from build123d import *

# Parameters (mm, degrees)
SKETCH1_W                = 98
SKETCH1_H                = 63
BOSS_EXTRUDE1_DEPTH      = 12
CUT_EXTRUDE1_REACH       = 61.475
SKETCH2_R                = 10
SKETCH2_R_2              = 6.5
SKETCH2_R_3              = 2.5
CUT_EXTRUDE2_REACH       = 61.475
SKETCH3_W                = 34
SKETCH3_H                = 12
F_5_0_5_DIAMETER_HOLE1_D = 5
CUT_EXTRUDE3_REACH       = 61.475
SKETCH11_W               = 25
SKETCH11_H               = 16
CUT_EXTRUDE4_REACH       = 61.475
FILLET1_R                = 2
CUT_EXTRUDE7_DEPTH       = 8
CUT_EXTRUDE8_DEPTH       = 6.5


with BuildPart() as part:
    # Sketch1 → Boss-Extrude1 (new body)
    with BuildSketch(Plane(origin=(0, 0, 0), x_dir=(1, 0, 0), z_dir=(0, 1, 0))):
        Rectangle(SKETCH1_W, SKETCH1_H)
    extrude(amount=BOSS_EXTRUDE1_DEPTH)

    # Sketch2 → Cut-Extrude1 (cut, up to next)
    with BuildSketch(Plane(origin=(0, 12, 0), x_dir=(1, 0, 0), z_dir=(0, 1, 0)), mode=Mode.PRIVATE) as cut_extrude1_sk1:
        with Locations(Location((0, 16.5, 0), (0, 0, 270))):
            Circle(SKETCH2_R)
    cut_extrude1_tool1 = extrude(cut_extrude1_sk1.sketch, amount=-CUT_EXTRUDE1_REACH, mode=Mode.PRIVATE) & part.part
    # Sketch2 → Cut-Extrude1 (cut, up to next)
    with BuildSketch(Plane(origin=(0, 12, 0), x_dir=(1, 0, 0), z_dir=(0, 1, 0)), mode=Mode.PRIVATE) as cut_extrude1_sk2:
        with Locations(Location((-28, -4.5, 0), (0, 0, 270))):
            Circle(SKETCH2_R_2)
    cut_extrude1_tool2 = extrude(cut_extrude1_sk2.sketch, amount=-CUT_EXTRUDE1_REACH, mode=Mode.PRIVATE) & part.part
    # Sketch2 → Cut-Extrude1 (cut, up to next)
    with BuildSketch(Plane(origin=(0, 12, 0), x_dir=(1, 0, 0), z_dir=(0, 1, 0)), mode=Mode.PRIVATE) as cut_extrude1_sk3:
        with Locations(Location((28, -4.5, 0), (0, 0, 270))):
            Circle(SKETCH2_R_2)
    cut_extrude1_tool3 = extrude(cut_extrude1_sk3.sketch, amount=-CUT_EXTRUDE1_REACH, mode=Mode.PRIVATE) & part.part
    # Sketch2 → Cut-Extrude1 (cut, up to next)
    with BuildSketch(Plane(origin=(0, 12, 0), x_dir=(1, 0, 0), z_dir=(0, 1, 0)), mode=Mode.PRIVATE) as cut_extrude1_sk4:
        with Locations(Location((-15, 16.5, 0), (0, 0, 270))):
            Circle(SKETCH2_R_3)
    cut_extrude1_tool4 = extrude(cut_extrude1_sk4.sketch, amount=-CUT_EXTRUDE1_REACH, mode=Mode.PRIVATE) & part.part
    # Sketch2 → Cut-Extrude1 (cut, up to next)
    with BuildSketch(Plane(origin=(0, 12, 0), x_dir=(1, 0, 0), z_dir=(0, 1, 0)), mode=Mode.PRIVATE) as cut_extrude1_sk5:
        with Locations(Location((15, 16.5, 0), (0, 0, 270))):
            Circle(SKETCH2_R_3)
    cut_extrude1_tool5 = extrude(cut_extrude1_sk5.sketch, amount=-CUT_EXTRUDE1_REACH, mode=Mode.PRIVATE) & part.part
    add(cut_extrude1_tool1.solids().sort_by_distance((0, 12, -16.5))[0], mode=Mode.SUBTRACT)
    add(cut_extrude1_tool2.solids().sort_by_distance((-28, 12, 4.5))[0], mode=Mode.SUBTRACT)
    add(cut_extrude1_tool3.solids().sort_by_distance((28, 12, 4.5))[0], mode=Mode.SUBTRACT)
    add(cut_extrude1_tool4.solids().sort_by_distance((-15, 12, -16.5))[0], mode=Mode.SUBTRACT)
    add(cut_extrude1_tool5.solids().sort_by_distance((15, 12, -16.5))[0], mode=Mode.SUBTRACT)

    # Sketch3 → Cut-Extrude2 (cut, up to next)
    with BuildSketch(Plane(origin=(0, 12, 0), x_dir=(1, 0, 0), z_dir=(0, 1, 0)), mode=Mode.PRIVATE) as cut_extrude2_sk1:
        with Locations((0, -25.5)):
            Rectangle(SKETCH3_W, SKETCH3_H)
    cut_extrude2_tool1 = extrude(cut_extrude2_sk1.sketch, amount=-CUT_EXTRUDE2_REACH, mode=Mode.PRIVATE) & part.part
    add(cut_extrude2_tool1.solids().sort_by_distance((0, 12, 25.5))[0], mode=Mode.SUBTRACT)

    # Ø5.0 (5) Diameter Hole1 (through all)
    with Locations(Plane(origin=(0, 12, 0), x_dir=(-1, 0, 0), z_dir=(0, 1, 0))):
        with Locations((28, 23.5), (-28, 23.5)):
            Hole(F_5_0_5_DIAMETER_HOLE1_D / 2)

    # Sketch11 → Cut-Extrude3 (cut, up to next)
    with BuildSketch(Plane(origin=(0, 12, 0), x_dir=(-1, 0, 0), z_dir=(0, 1, 0)), mode=Mode.PRIVATE) as cut_extrude3_sk1:
        with Locations((36.5, -23.5)):
            Rectangle(SKETCH11_W, SKETCH11_H)
    cut_extrude3_tool1 = extrude(cut_extrude3_sk1.sketch, amount=-CUT_EXTRUDE3_REACH, mode=Mode.PRIVATE) & part.part
    cut_extrude3 = cut_extrude3_tool1.solids().sort_by_distance((-36.5, 12, -23.5))[0]
    add(cut_extrude3, mode=Mode.SUBTRACT)

    # Mirror1: Cut-Extrude3 across plane
    add(cut_extrude3.mirror(Plane(origin=(0, 0, 0), x_dir=(0, 0, 1), z_dir=(1, 0, 0))), mode=Mode.SUBTRACT)

    # Sketch12 → Cut-Extrude4 (cut, up to next)
    with BuildSketch(Plane(origin=(0, 12, 0), x_dir=(1, 0, 0), z_dir=(0, 1, 0)), mode=Mode.PRIVATE) as cut_extrude4_sk1:
        with BuildLine():
            Line((-17, -19.5), (-13, -19.5))
            ThreePointArc((-13, -19.5), (-15, -17.5), (-17, -19.5))
        make_face()
    cut_extrude4_tool1 = extrude(cut_extrude4_sk1.sketch, amount=-CUT_EXTRUDE4_REACH, mode=Mode.PRIVATE) & part.part
    # Sketch12 → Cut-Extrude4 (cut, up to next)
    with BuildSketch(Plane(origin=(0, 12, 0), x_dir=(1, 0, 0), z_dir=(0, 1, 0)), mode=Mode.PRIVATE) as cut_extrude4_sk2:
        with BuildLine():
            Line((13, -19.5), (17, -19.5))
            ThreePointArc((17, -19.5), (15, -17.5), (13, -19.5))
        make_face()
    cut_extrude4_tool2 = extrude(cut_extrude4_sk2.sketch, amount=-CUT_EXTRUDE4_REACH, mode=Mode.PRIVATE) & part.part
    add(cut_extrude4_tool1.solids().sort_by_distance((-15, 12, 18.651174))[0], mode=Mode.SUBTRACT)
    add(cut_extrude4_tool2.solids().sort_by_distance((15, 12, 18.651174))[0], mode=Mode.SUBTRACT)

    # Fillet1
    fillet1_edges = [part.edges().sort_by_distance(p)[0] for p in [
        (-49, 6, -15.5),
        (-24, 6, -31.5),
        (-24, 6, -15.5),
        (49, 6, -15.5),
        (24, 6, -15.5),
        (24, 6, -31.5),
    ]]
    fillet(fillet1_edges, radius=FILLET1_R)

    # Sketch18 → Cut-Extrude7 (cut)
    with BuildSketch(Plane(origin=(-30.447133355, 0, 87.682451642), x_dir=(1, 0, 0), z_dir=(0, -1, 0))):
        with BuildLine():
            Line((26.447133355, -78.182451642), (34.447133355, -78.182451642))
            ThreePointArc((34.447133355, -78.182451642), (36.447133355, -80.182451642), (34.447133355, -82.182451642))
            Line((34.447133355, -82.182451642), (26.447133355, -82.182451642))
            ThreePointArc((26.447133355, -82.182451642), (24.447133355, -80.182451642), (26.447133355, -78.182451642))
        make_face()
    extrude(amount=-CUT_EXTRUDE7_DEPTH, mode=Mode.SUBTRACT)

    # Sketch20 → Cut-Extrude8 (cut)
    with BuildSketch(Plane(origin=(-30.447133355, 0, 87.682451642), x_dir=(1, 0, 0), z_dir=(0, -1, 0))):
        with BuildLine():
            Line((32.947133355, -47.95431377), (32.947133355, -85.182451642))
            ThreePointArc((32.947133355, -85.182451642), (30.447133355, -87.682451642), (27.947133355, -85.182451642))
            Line((27.947133355, -85.182451642), (27.947133355, -47.95431377))
            ThreePointArc((27.947133355, -47.95431377), (30.447133355, -45.45431377), (32.947133355, -47.95431377))
        make_face()
    extrude(amount=-CUT_EXTRUDE8_DEPTH, mode=Mode.SUBTRACT)


solid = part.part
CAD build for the part. Positions are in the model's coordinates, mm. A direction names the side the tool comes from. Coordinates: 2 decimals unless noted, no trailing zeros. Write each loop counter-clockwise with the first axis right and the second up, starting at its lowest first coordinate (ties: lowest second). Pieces come first, ordered by that corner, then holes. Notation, with made-up numbers: (80, 70) - (115, 70) arc R24 ccw to (115, 85) - close; hole circle Ø4 at (-31.5, -36). An arc over 180 degrees is marked (long way). Use a Markdown table: item, result. Add a question column.
Item 1: Band-saw the part on B-B, the plane z = 7.5. Give the cut face in (x, y).
Item 2: Band-saw the part on C-C, the plane x = -28. Give the cut face in (y, z).
Item 3: Band-saw the part on A-A, the plane x = -15. Give the cut face in (y, z).
Item 4: Flat gauge pins, fed straight in: pin 1 (6 mm diameter, centred on x = -28, z = 23.5, fed in from -Y); pin 2 (6 mm diameter, centred on y = 8.5, z = -23.5, fed in from +X); pin 3 (3.5 mm diameter, centred on y = 9, z = -22, fed in from -X); pin 4 (4 mm diameter, centred on x = -15, z = -16.5, fed in from -Y). Where does each tip first touch, or does it go through?
Item 5: 3-axis set-ups, long thin cutter, end or side, ignore diameter. For faces 1 (the face through (17, 6, 26)), 2 (the face through (36, 6, -15.5)), 3 (the face through (0, 6.5, 3)), 4 (the face through (-36, 6, -15.5)): which of +Z, -Z, +X, -X, +Y, -Y reach the whole face in a straight line?
Item 6: Band-saw the part on D-D, the plane z = -16.5. Give the cut face in (x, y).
Item 7: Mould opens along Z. For faces 5 (the face through (15, 6.1, 17.5)), 6 (the face through (13, 6, -18)), 7 (the face through (0, 6, -31.5)) say: pulls with the +Z half, pulls with the -Z half, needs draft (parallel to the pull), parting line crosses it, or undercut.
Item 8: Drill centre lines: L1, parallel to X at y = 2.5, z = 4.5; L2, parallel to X at y = 3.5, z = -18; L3, parallel to Z at x = 26.5, y = 5. Where is each one in solid material? Low to high. Write a range as from..to.
Numbers:
| question | item | result |
|---|---|---|
| 1 | outline | (-49, 0) - (-33.77, 0) - (-33.77, 12) - (-49, 12) - close; (-22.23, 0) - (-6, 0) - (-6, 8) - (6, 8) - (6, 0) - (22.23, 0) - (22.23, 12) - (-22.23, 12) - close; (33.77, 0) - (49, 0) - (49, 12) - (33.77, 12) - close |
| 2 | outline | (0, -15.5) - (12, -15.5) - (12, -2) - (0, -2) - close; (0, 11) - (12, 11) - (12, 21) - (0, 21) - close; (0, 26) - (12, 26) - (12, 31.5) - (0, 31.5) - close |
| 3 | outline | (0, -31.5) - (12, -31.5) - (12, -19) - (0, -19) - close; (0, -14) - (12, -14) - (12, 17.5) - (0, 17.5) - close |
| 4 | pin 1 | y = 0 |
| 4 | pin 2 | x = 24 |
| 4 | pin 3 | x = -24 |
| 4 | pin 4 | through |
| 5 | face 1 | +Z, +Y, -Y |
| 5 | face 2 | -Z, +X, +Y, -Y |
| 5 | face 3 | +Z, -Y |
| 5 | face 4 | -Z, -X, +Y, -Y |
| 6 | outline | (-24.27, 0) - (-17.5, 0) - (-17.5, 12) - (-24.27, 12) - close; (-12.5, 0) - (-10, 0) - (-10, 12) - (-12.5, 12) - close; (10, 0) - (12.5, 0) - (12.5, 12) - (10, 12) - close; (17.5, 0) - (24.27, 0) - (24.27, 12) - (17.5, 12) - close |
| 7 | face 5 | pulls with the +Z half |
| 7 | face 6 | undercut |
| 7 | face 7 | pulls with the -Z half |
| 8 | L1 | -49..-34.5, -21.5..-2.5, 2.5..21.5, 34.5..49 |
| 8 | L2 | -24..-17, -13..-9.89, 9.89..13, 17..24 |
| 8 | L3 | -15.5..-1.82, 10.82..21.5, 25.5..31.5 |
